from build123d import *

# Parameters (mm, degrees)
F0_R     = 7.9375
F1_DEPTH = 6.35


with BuildPart() as f1:
    # F0 (on Front) → F1 (new body)
    with BuildSketch(Plane.XZ):
        Polygon((63.5, 0), (63.5, 41.275), (0, 28.575), (0, 0), align=None)
        with Locations((12.7, 15.875)):
            Circle(F0_R, mode=Mode.SUBTRACT)
    extrude(amount=-F1_DEPTH)


solid = f1.part
Here's how the part is built. I have some questions about the finished solid (model axes, mm). Give positions to 0.01 mm unless a question says otherwise; leave off trailing zeros. Order: outer loops, then holes, each group sorted by start corner. A loop starts at its lowest first (then second) coordinate and runs counter-clockwise, first axis right, second up. Notation, with made-up numbers: M 80.5,-11 L 99.5,-11 A26 ccw 99.5,16 Z; hole C 59,54 d8. An arc over 180 degrees is marked long. Answer as a JSON object with one key per item and string values. Group by question number.
1) Suppose I cut it at C-C, the plane z = 32. Write out the boundary of the cut face in (x, y) (3 decimals).
2) Suppose I cut it at D-D, the plane x = 52.5. Write out the boundary of the cut face in (y, z) (3 decimals).
3) We'd pull the mould along X, two halves only. Please class faces 1 (the flat face through (31, 3, 0)), 2 (the flat face through (63.5, 3, 20)), 3 (the flat face through (32.194, 3.131, 35.014)), 4 (the cylindrical face through (20.27, 3.13, 18.26)): pulls with the +X half, pulls with the -X half, needs draft (parallel to the pull), parting line crosses it, or undercut.
4) Please list where these lines run through material, in increasing order: L1, parallel to X at y = 1.5, z = 18; L2, parallel to Z at x = 12.7, y = 2.25 (1 decimal); L3, parallel to X at y = 2.75, z = 12.5. Write a range as [from, to].
5) I'm going to push a flat-ended pin straight in: pin 1 Ø3 at (x, z) = (7, 18.5) entering from -Y. Where does the tip first touch, or does it pass through?
6) Suppose I cut it at B-B, the plane y = 2. Write out the boundary of the cut face in (x, z) (1 decimal), plus the area to 3 significant figures.
Results found:
{
 "1": {"outline": "M 17.125,0 L 63.5,0 L 63.5,6.35 L 17.125,6.35 Z"},
 "2": {"outline": "M 0,0 L 6.35,0 L 6.35,39.075 L 0,39.075 Z"},
 "3": {"face 1": "needs draft", "face 2": "pulls with the +X half", "face 3": "pulls with the -X half", "face 4": "undercut"},
 "4": {"L1": "[0, 5.05], [20.35, 63.5]", "L2": "[0, 7.9], [23.8, 31.1]", "L3": "[0, 5.52], [19.88, 63.5]"},
 "5": {"pin 1": "through"},
 "6": {"outline": "M 0,0 L 63.5,0 L 63.5,41.3 L 0,28.6 Z; hole C 12.7,15.9 d15.9", "area": "2,020 mm²"}
}
